Read the model definition and answer for the solid it produces. Units are mm, in the model's axes. Face numbers are marked on the shaded views. A direction names the side the tool comes from. Round coordinates to 2 decimals unless told otherwise and drop trailing zeros. Order: outer loops, then holes, each group sorted by start corner. A loop starts at its lowest first (then second) coordinate and runs counter-clockwise, first axis right, second up. Notation, with made-up numbers: (61, 45) -> (108, 45) arc R12 ccw to (108, 55) -> close; hole circle Ø6 at (38.25, -19). An arc over 180 degrees is marked (long way). Use a Markdown table: item, result. Add a question column.
1. Section C-C, the plane x = 0 is taken. Give the vertices of the cut face in (y, z), then the cut area to 3 significant figures.
2. Consider L1, parallel to X at y = 10.75, z = -6; L2, parallel to Z at x = 0, y = -2.8; L3, parallel to Z at x = 11.5, y = 10. Determine where each line is inside the solid, lowest interval first. Write a range as [from, to].
3. Section B-B, the plane z = 0 is taken. Give the vertices of the cut face in (x, y), then the cut area to 3 significant figures.
4. The mould has two halves that part along X. Classify the marked faces 4, 5 and 6: +X half, -X half, draft (parallel to the pull), parting line (faces both ways), or undercut.
5. Section D-D, the plane z = 8.25 is taken. Give the vertices of the cut face in (x, y), then the cut area to 3 significant figures.
6. Section A-A, the plane y = 10.5 is taken. Give the vertices of the cut face in (x, z).
7. For the marked faces 1, 2 and 3, determine the directions among +Z, -Z, +X, -X, +Y, -Y from which every point of the face is accessible in a straight line to the end or side of a thin tool.
8. Given pin 1 (0.6 mm diameter, centred on x = 11, z = 0.5, fed in from +Y); pin 2 (1 mm diameter, centred on x = -9.5, y = 9.5, fed in from -Z), each flat-ended and moving along its own axis, determine where each tip first touches the part or whether it passes through.
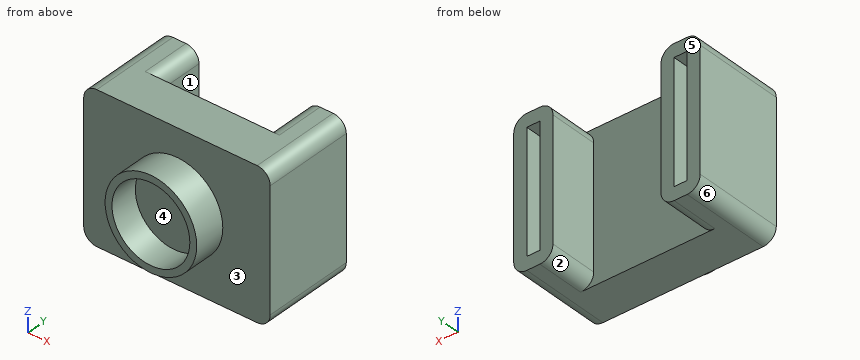
Autodesk Inventor part; units mm, degrees
ref_plane "YZ Plane" through (0, 0, 0) normal (1, 0, 0) x (0, 1, 0)
ref_plane "XZ Plane" through (0, 0, 0) normal (0, 1, 0) x (-1, 0, 0)
ref_plane "XY Plane" through (0, 0, 0) normal (0, 0, 1) x (1, 0, 0)
sketch "Sketch1" plane through (0, 0, 0) normal (0, 0, 1) x (1, 0, 0)
  line L0 (0, 0) -> (7, 0)
  line L1 (7, 0) -> (7, 7)
  line L2 (7, 7) -> (0, 7)
  line L3 (0, 7) -> (0, 0)
  line L4 (7, 0) -> (5.95, 0)
  line L5 (5.95, 0) -> (5.95, -4.3)
  line L6 (5.95, -4.3) -> (7, -4.3)
  line L7 (7, -4.3) -> (7, 0)
  dimension "d0" = 7
  dimension "d1" = 7
  dimension "d2" = 1.05
  dimension "d3" = 4.3
revolve "Revolution1" add sketch "Sketch1" angle 360 about axis through (0, 7, 0) along (0, -1, 0)
sketch "Sketch2" plane through (0, 7, 0) normal (0, 1, 0) x (1, 0, 0)
  line L0 (-14.25, -11.25) -> (14.25, -11.25)
  line L1 (14.25, -11.25) -> (14.25, 11.25)
  line L2 (14.25, 11.25) -> (-14.25, 11.25)
  line L3 (-14.25, 11.25) -> (-14.25, -11.25)
  line L4 (-14.25, -11.25) -> (14.25, 11.25) construction
  line L5 (14.25, -11.25) -> (-14.25, 11.25) construction
  point P0 (0, 0)
  dimension "d5" = 28.5
  dimension "d6" = 22.5
extrude "Extrusion1" add sketch "Sketch2" against normal blind 6.5
fillet "Fillet1" radius 2 4 edges at (-14.25, 3.75, 11.25) (-14.25, 3.75, -11.25) (14.25, 3.75, 11.25) (14.25, 3.75, -11.25)
sketch "Sketch3" plane through (-12.25, 7, -11.25) normal (0, 1, 0) x (1, 0, 0)
  arc A0 (26.5, -2) -> (24.5, 0) centre (24.5, -2) ccw
  line L0 (24.5, 0) -> (0, 0)
  arc A1 (0, 0) -> (-2, -2) centre (0, -2) ccw
  line L1 (-2, -2) -> (-2, -20.5)
  arc A2 (-2, -20.5) -> (0, -22.5) centre (0, -20.5) ccw
  line L2 (0, -22.5) -> (24.5, -22.5)
  arc A3 (24.5, -22.5) -> (26.5, -20.5) centre (24.5, -20.5) ccw
  line L3 (26.5, -20.5) -> (26.5, -2)
  line L4 (24.5, 0) -> (0, 0)
  line L5 (0, -22.5) -> (2, -22.5)
  line L6 (4, -20.5) -> (4, -2)
  line L7 (2, 0) -> (0, 0)
  line L8 (-2, -2) -> (-2, -20.5)
  arc A4 (0, 0) -> (-2, -2) centre (0, -2) ccw
  arc A5 (4, -2) -> (2, 0) centre (2, -2) ccw
  arc A6 (-2, -20.5) -> (0, -22.5) centre (0, -20.5) ccw
  arc A7 (2, -22.5) -> (4, -20.5) centre (2, -20.5) ccw
  line L9 (12.25, 1.2488) -> (12.25, 2.7237)
  arc A8 (26.5, -2) -> (24.5, 0) centre (24.5, -2) ccw
  line L10 (26.5, -2) -> (26.5, -20.5)
  arc A9 (24.5, -22.5) -> (26.5, -20.5) centre (24.5, -20.5) ccw
  line L11 (24.5, -22.5) -> (22.5, -22.5)
  line L12 (20.5, -20.5) -> (20.5, -2)
  line L13 (22.5, 0) -> (24.5, 0)
  line L14 (26.5, -2) -> (26.5, -20.5)
  arc A10 (26.5, -2) -> (24.5, 0) centre (24.5, -2) ccw
  arc A11 (22.5, 0) -> (20.5, -2) centre (22.5, -2) ccw
  arc A12 (24.5, -22.5) -> (26.5, -20.5) centre (24.5, -20.5) ccw
  arc A13 (20.5, -20.5) -> (22.5, -22.5) centre (22.5, -20.5) ccw
  line L15 (2, -2) -> (2, -20.5)
  line L16 (2, -20.5) -> (0, -20.5)
  line L17 (0, -20.5) -> (0, -2)
  line L18 (0, -2) -> (2, -2)
  line L19 (22.5, -2) -> (22.5, -20.5)
  line L20 (22.5, -20.5) -> (24.5, -20.5)
  line L21 (24.5, -20.5) -> (24.5, -2)
  line L22 (24.5, -2) -> (22.5, -2)
  point P0 (12.25, -11.25)
  point P1 (4, 0)
  point P2 (-2, 0)
  point P3 (20.5, 0)
  point P4 (26.5, 0)
  point P5 (2, 0)
  point P6 (2, -22.5)
  dimension "d10" = 6
  dimension "d11" = 2
  dimension "d12" = 2
  dimension "d13" = 2
extrude "Extrusion2" add sketch "Sketch3" along normal blind 7.5 contours L3 A3 L2 A13 L12 A11 L0 A0 | A5 L6 A7 L2 A2 L1 A1 L0
properties part number "Keller"
Verdict:
| question | item | result |
|---|---|---|
| 1 | outline | (-4.3, -7) -> (0.5, -7) -> (0.5, -11.25) -> (7, -11.25) -> (7, 11.25) -> (0.5, 11.25) -> (0.5, 7) -> (-4.3, 7) -> (-4.3, 5.95) -> (0, 5.95) -> (0, -5.95) -> (-4.3, -5.95) -> close |
| 1 | area | 162 mm2 |
| 2 | L1 | x = [-14.25, -12.25], [-10.25, -8.25], [8.25, 10.25], [12.25, 14.25] |
| 2 | L2 | z = [-7, -5.95], [5.95, 7] |
| 2 | L3 | z = [-11.25, -9.25], [9.25, 11.25] |
| 3 | outline | (-14.25, 0.5) -> (-7, 0.5) -> (-7, -4.3) -> (-5.95, -4.3) -> (-5.95, 0) -> (5.95, 0) -> (5.95, -4.3) -> (7, -4.3) -> (7, 0.5) -> (14.25, 0.5) -> (14.25, 14.5) -> (12.25, 14.5) -> (12.25, 7) -> (10.25, 7) -> (10.25, 14.5) -> (8.25, 14.5) -> (8.25, 7) -> (-8.25, 7) -> (-8.25, 14.5) -> (-10.25, 14.5) -> (-10.25, 7) -> (-12.25, 7) -> (-12.25, 14.5) -> (-14.25, 14.5) -> close |
| 3 | area | 261 mm2 |
| 4 | face 4 | undercut |
| 4 | face 5 | draft |
| 4 | face 6 | -X half |
| 5 | outline | (-14.25, 0.5) -> (14.25, 0.5) -> (14.25, 14.5) -> (12.25, 14.5) -> (12.25, 7) -> (10.25, 7) -> (10.25, 14.5) -> (8.25, 14.5) -> (8.25, 7) -> (-8.25, 7) -> (-8.25, 14.5) -> (-10.25, 14.5) -> (-10.25, 7) -> (-12.25, 7) -> (-12.25, 14.5) -> (-14.25, 14.5) -> close |
| 5 | area | 245 mm2 |
| 6 | outline | (-14.25, -9.25) arc R2 ccw to (-12.25, -11.25) -> (-10.25, -11.25) arc R2 ccw to (-8.25, -9.25) -> (-8.25, 9.25) arc R2 ccw to (-10.25, 11.25) -> (-12.25, 11.25) arc R2 ccw to (-14.25, 9.25) -> close; (8.25, -9.25) arc R2 ccw to (10.25, -11.25) -> (12.25, -11.25) arc R2 ccw to (14.25, -9.25) -> (14.25, 9.25) arc R2 ccw to (12.25, 11.25) -> (10.25, 11.25) arc R2 ccw to (8.25, 9.25) -> close; hole (-12.25, -9.25) -> (-10.25, -9.25) -> (-10.25, 9.25) -> (-12.25, 9.25) -> close; hole (10.25, -9.25) -> (12.25, -9.25) -> (12.25, 9.25) -> (10.25, 9.25) -> close |
| 7 | face 1 | +Z, -Z, +Y |
| 7 | face 2 | -Z, +Y |
| 7 | face 3 | -Y |
| 8 | pin 1 | stops at y = 7 |
| 8 | pin 2 | stops at z = -11.23 |
